Geometry check sheet. Reference: the model listing, model coordinates, mm. Round coordinates to 2 decimals unless told otherwise and drop trailing zeros. Write each loop counter-clockwise with the first axis right and the second up, starting at its lowest first coordinate (ties: lowest second). Pieces come first, ordered by that corner, then holes.
from build123d import *

# Parameters (mm, degrees)
SKETCH1_W           = 33.02
SKETCH1_H           = 20.32
SKETCH1_R           = 3.3
BOSS_EXTRUDE1_DEPTH = 3.175
SKETCH2_R           = 1.1303
CUT_EXTRUDE1_DEPTH  = 39.901200817


with BuildPart() as part:
    # Sketch1 → Boss-Extrude1 (new body)
    with BuildSketch(Plane(origin=(0, 0, 0), x_dir=(1, 0, 0), z_dir=(0, 1, 0))):
        with Locations((16.51, 10.16)):
            Rectangle(SKETCH1_W, SKETCH1_H)
        with Locations(Location((23.02, 7.5, 0), (0, 0, 270))):
            Circle(SKETCH1_R, mode=Mode.SUBTRACT)
    extrude(amount=BOSS_EXTRUDE1_DEPTH)

    # Sketch2 → Cut-Extrude1 (cut, through all)
    with BuildSketch(Plane(origin=(0, 3.175, 0), x_dir=(1, 0, 0), z_dir=(0, 1, 0))):
        with Locations(Location((7.78, 5.1562, 0), (0, 0, 270))):
            Circle(SKETCH2_R)
        with Locations(Location((7.78, 14.6812, 0), (0, 0, 270))):
            Circle(SKETCH2_R)
    extrude(amount=-CUT_EXTRUDE1_DEPTH, mode=Mode.SUBTRACT)


solid = part.part
1. Section check A-A (x = 23.02). Record the cut outline in (y, z) (3 decimals), plus the area to 3 significant figures.
2. Section check C-C (x = 7.78). Record the cut outline in (y, z) (1 decimal).
3. Section check B-B (z = -7.5). Record the cut outline in (x, y) (3 decimals).
4. Scan lines: line 1 along X through (y, z) = (1.65, -5); line 2 along X through (y, z) = (2.2, -7.5); line 3 along Z through (x, y) = (23, 2.5). Record each from-to range of solid material in increasing order.
5. Release check for a two-part mould opening along X. For faces 1 (the face through (33.02, 2, -10)), 2 (the face through (19.8, 1.57, -8.22)), 3 (the face through (0, 2, -10)), 4 (the face through (16, 2, 0)) record: +X half, -X half, draft (parallel to the pull), parting line (faces both ways), or undercut.
6. Section check D-D (y = 1.85). Record the cut outline in (x, z).
Results below:
1. outline: (0, -20.32) - (3.175, -20.32) - (3.175, -10.8) - (0, -10.8) - close; (0, -4.2) - (3.175, -4.2) - (3.175, 0) - (0, 0) - close
1. area: 43.6 mm2
2. outline: (0, -20.3) - (3.2, -20.3) - (3.2, -15.8) - (0, -15.8) - close; (0, -13.6) - (3.2, -13.6) - (3.2, -6.3) - (0, -6.3) - close; (0, -4) - (3.2, -4) - (3.2, 0) - (0, 0) - close
3. outline: (0, 0) - (19.72, 0) - (19.72, 3.175) - (0, 3.175) - close; (26.32, 0) - (33.02, 0) - (33.02, 3.175) - (26.32, 3.175) - close
4. line 1: x = 0 to 6.66, 8.9 to 20.87, 25.17 to 33.02
4. line 2: x = 0 to 19.72, 26.32 to 33.02
4. line 3: z = -20.32 to -10.8, -4.2 to 0
5. face 1: +X half
5. face 2: undercut
5. face 3: -X half
5. face 4: draft
6. outline: (0, -20.32) - (33.02, -20.32) - (33.02, 0) - (0, 0) - close; hole circle Ø2.26 at (7.78, -14.68); hole circle Ø2.26 at (7.78, -5.16); hole circle Ø6.6 at (23.02, -7.5)
